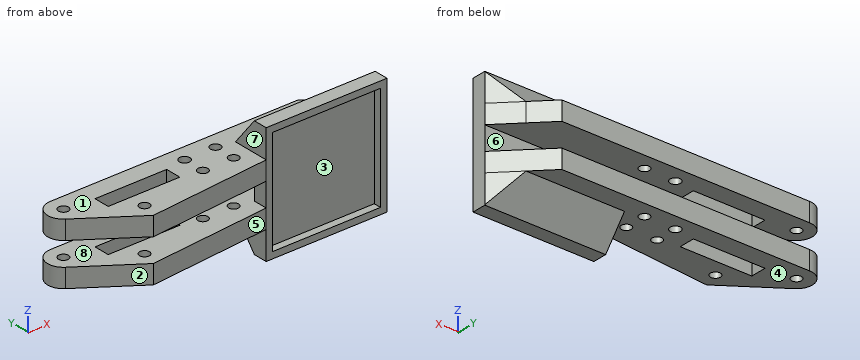
```python
from build123d import *

# Parameters (mm, degrees)
RESSALTO_EXTRUS_O1_DEPTH         = 8
RESSALTO_EXTRUS_O2_DEPTH         = 51.268117765
CORTE_EXTRUS_O1_DEPTH            = 8.000000002
ESBO_O4_W                        = 51.268117776
ESBO_O4_H                        = 10.000000011
CORTE_EXTRUS_O2_DEPTH            = 17.723100001
CORTE_EXTRUS_O3_DEPTH            = 40.852574409
ESBO_O6_W                        = 51.268117776
ESBO_O6_H                        = 10.000000011
CORTE_EXTRUS_O4_DEPTH            = 0.151992449
RESSALTO_EXTRUS_O3_START         = 7.999999998
RESSALTO_EXTRUS_O3_DEPTH         = 7.999999998
RESSALTO_EXTRUS_O4_DEPTH         = 12.017232655
RESSALTO_EXTRUS_O5_DEPTH         = 12.017232657
ESBO_O10_W                       = 30.391419991
ESBO_O10_H                       = 6.689959998
CORTE_EXTRUS_O5_DEPTH            = 135.855194678
ESBO_O11_W                       = 30.391419991
ESBO_O11_H                       = 6.689959998
CORTE_EXTRUS_O6_DEPTH            = 135.855194677
ESBO_O12_W                       = 45.768117767
ESBO_O12_H                       = 44.53446532
CORTE_EXTRUS_O7_DEPTH            = 3.15
INCLINA_O1_START                 = 9.762479363
INCLINA_O1_DEPTH                 = 8.237520637
INCLINA_O2_START                 = -6.465378083
INCLINA_O2_DEPTH                 = 8.465378083
INCLINA_O3_ANGLE                 = 84.752120974
FURO_COM_FOLGA_DE_M41_D          = 4.452840696
FURO_COM_FOLGA_DE_M41_DEPTH      = 7.999999998
FURO_DE_DI_METRO_4_2_4_2_1_D     = 4.2
FURO_DE_DI_METRO_4_2_4_2_1_DEPTH = 7.999999998
FURO_COM_FOLGA_DE_M42_D          = 4.452840696
FURO_COM_FOLGA_DE_M42_DEPTH      = 38.017232657
FURO1_D                          = 4.246430182
FURO1_DEPTH                      = 38.017232657


with BuildPart() as part:
    # Esboço1 → Ressalto-extrusão1 (new body)
    with BuildSketch(Plane.XY.offset(8)):
        with BuildLine():
            Line((-36.110267765, -64.727666859), (-36.110267765, 0))
            Line((-36.110267765, 0), (-107.75607805, 0))
            ThreePointArc((-107.75607805, 0), (-114.12766225, -4.677735132), (-111.573397577, -12.157977319))
            Line((-111.573397577, -12.157977319), (-36.110267765, -64.727666859))
        make_face()
    extrude(amount=-RESSALTO_EXTRUS_O1_DEPTH)

    # Esboço2 → Ressalto-extrusão2 (add)
    with BuildSketch(Plane(origin=(-36.110267765, 0, 0), x_dir=(0, 0, -1), z_dir=(1, 0, 0))):
        with BuildLine():
            Line((2e-09, 1e-09), (2e-09, -23.87509245))
            add(Edge.make_bspline(
                [(2e-09, -64.727666859), (2e-09, -51.110142056), (2e-09, -37.492617253), (2e-09, -23.87509245)],
                knots=[0, 0, 0, 0, 1, 1, 1, 1], degree=3))
            Line((2e-09, -64.727666859), (-18.000000002, -64.727666859))
            add(Edge.make_bspline(
                [(-18.000000002, -64.727666859), (-18.000000002, -51.110142056), (-18.000000002, -37.492617253), (-18.000000002, -23.87509245)],
                knots=[0, 0, 0, 0, 1, 1, 1, 1], degree=3))
            Line((-18.000000002, -23.87509245), (-18.000000002, -17.875092449))
            add(Edge.make_bspline(
                [(-18.000000002, -17.723099999), (-18.000000002, -17.773764149), (-18.000000002, -17.824428299), (-18.000000002, -17.875092449)],
                knots=[0, 0, 0, 0, 1, 1, 1, 1], degree=3))
            add(Edge.make_bspline(
                [(-18.000000002, 1e-09), (-18.000000002, -5.907699999), (-18.000000002, -11.815399999), (-18.000000002, -17.723099999)],
                knots=[0, 0, 0, 0, 1, 1, 1, 1], degree=3))
            Line((-18.000000002, 1e-09), (2e-09, 1e-09))
        make_face()
    extrude(amount=RESSALTO_EXTRUS_O2_DEPTH)

    # Esboço3 → Corte-extrusão1 (cut)
    with BuildSketch(Plane(origin=(0, 0, 0), x_dir=(-1, 0, 0), z_dir=(0, 0, -1))):
        Polygon((-15.15785, 0), (-15.15785, -17.7231), (2.585682, 0), align=None)
    extrude(amount=-CORTE_EXTRUS_O1_DEPTH, mode=Mode.SUBTRACT)

    # Esboço4 → Corte-extrusão2 (cut)
    with BuildSketch(Plane(origin=(0, 0, 0), x_dir=(-1, 0, 0), z_dir=(0, 1, 0))):
        with Locations((10.476208888, 13.000000002)):
            Rectangle(ESBO_O4_W, ESBO_O4_H)
    extrude(amount=-CORTE_EXTRUS_O2_DEPTH, mode=Mode.SUBTRACT)

    # Esboço5 → Corte-extrusão3 (cut)
    with BuildSketch(Plane.XZ.offset(64.727666859)):
        Polygon((15.15785, 18.000000002), (-36.110267765, 18.000000002), (-36.110267765, 8), (-36.110267765, -2e-09), (15.15785, -2e-09), align=None)
    extrude(amount=-CORTE_EXTRUS_O3_DEPTH, mode=Mode.SUBTRACT)

    # Esboço6 → Corte-extrusão4 (cut)
    with BuildSketch(Plane(origin=(0, -17.723100001, 0), x_dir=(-1, 0, 0), z_dir=(0, 1, 0))):
        with Locations((10.476208888, 13.000000002)):
            Rectangle(ESBO_O6_W, ESBO_O6_H)
    extrude(amount=-CORTE_EXTRUS_O4_DEPTH, mode=Mode.SUBTRACT)

    # Esboço7 → Ressalto-extrusão3 (add)
    with BuildSketch(Plane.XY.offset(18.000000002).offset(RESSALTO_EXTRUS_O3_START)):
        with BuildLine():
            Line((-36.110267767, -23.87509245), (-36.110267767, -64.727666793))
            Line((-36.110267767, -64.727666793), (-111.573397573, -12.157977315))
            ThreePointArc((-111.573397573, -12.157977315), (-114.127662248, -4.677735132), (-107.75607805, 1e-09))
            Line((-107.75607805, 1e-09), (-2.585681995, 1e-09))
            Line((-2.585681995, 1e-09), (5.698950337, -8.275092449))
            Line((5.698950337, -8.275092449), (15.157849978, -17.723100021))
            Line((15.157849978, -17.723100021), (15.157849978, -23.87509245))
            Line((15.157849978, -23.87509245), (-36.110267767, -23.87509245))
        make_face()
    extrude(amount=-RESSALTO_EXTRUS_O3_DEPTH)

    # Esboço8 → Ressalto-extrusão4 (add)
    with BuildSketch(Plane(origin=(0, 0, 0), x_dir=(-1, 0, 0), z_dir=(0, 0, -1))):
        Polygon((36.110267765, -8.275092449), (36.110267765, -23.87509245), (-15.15785, -23.87509245), (-15.15785, -17.7231), (-5.698950354, -8.275092449), align=None)
    extrude(amount=RESSALTO_EXTRUS_O4_DEPTH)

    # Esboço9 → Ressalto-extrusão5 (add)
    with BuildSketch(Plane.XY.offset(26)):
        Polygon((15.15785, -17.7231), (15.15785, -23.87509245), (-36.110267765, -23.87509245), (-36.110267765, -8.275092449), (5.698950354, -8.275092449), align=None)
    extrude(amount=RESSALTO_EXTRUS_O5_DEPTH)

    # Esboço10 → Corte-extrusão5 (cut, through all)
    with BuildSketch(Plane.XY.offset(8)):
        with Locations((-80.248070001, -11.317270001)):
            Rectangle(ESBO_O10_W, ESBO_O10_H)
    extrude(amount=-CORTE_EXTRUS_O5_DEPTH, mode=Mode.SUBTRACT)

    # Esboço11 → Corte-extrusão6 (cut, through all)
    with BuildSketch(Plane(origin=(0, 0, 18.000000002), x_dir=(-1, 0, 0), z_dir=(0, 0, -1))):
        with Locations((80.248070001, -11.317270001)):
            Rectangle(ESBO_O11_W, ESBO_O11_H)
    extrude(amount=-CORTE_EXTRUS_O6_DEPTH, mode=Mode.SUBTRACT)

    # Esboço12 → Corte-extrusão7 (cut)
    with BuildSketch(Plane.XZ.offset(23.87509245)):
        with Locations((-10.476208882, 13)):
            Rectangle(ESBO_O12_W, ESBO_O12_H)
    extrude(amount=-CORTE_EXTRUS_O7_DEPTH, mode=Mode.SUBTRACT)

    # Inclinação1: read off the stored shape, not the designer's step
    # Inclinação1 outline → Inclinação1 (cut)
    with BuildSketch(Plane(origin=(0, 0, 0), x_dir=(1, 0, 0), z_dir=(0, 0.7813058431702609, 0.624148363314371)).offset(INCLINA_O1_START)):
        Polygon((-36.110267765, -40.859795712), (15.15785, -40.859795712), (15.15785, -40.616276003), (5.698950337, -25.478837331), (-36.110267765, -25.478837331), align=None)
    extrude(amount=INCLINA_O1_DEPTH, mode=Mode.SUBTRACT)

    # Inclinação2: read off the stored shape, not the designer's step
    # Inclinação2 outline → Inclinação2 (cut)
    with BuildSketch(Plane(origin=(0, 0, 0), x_dir=(1, 0, 0), z_dir=(0, 0.7813058431702609, -0.624148363314371)).offset(INCLINA_O2_START)):
        Polygon((5.698950354, 5.164885408), (15.15785, 20.302324047), (15.15785, 20.545843787), (-36.110267765, 20.545843787), (-36.110267765, 5.164885408), align=None)
    extrude(amount=INCLINA_O2_DEPTH, mode=Mode.SUBTRACT)

    # Inclinação3
    inclina_o3_faces = [part.faces().sort_by_distance(p)[0] for p in [
        (-36.110267765, -44.301379654, 3.999999999),
        (-36.110267767, -44.301379621, 22.000000001),
    ]]
    draft(inclina_o3_faces, Plane(origin=(0, -23.87509245, 0), x_dir=(0, 0, -1), z_dir=(0, -1, 0)), INCLINA_O3_ANGLE)

    # Furo com folga de M41
    with Locations(Plane.XY.offset(26)):
        with Locations((-56.444514416, -6.798608997)):
            Hole(FURO_COM_FOLGA_DE_M41_D / 2, depth=FURO_COM_FOLGA_DE_M41_DEPTH)

    # Furo de diâmetro Ø4.2 (4.2)1
    with Locations(Plane.XY.offset(26)):
        with Locations((-85.990622049, -21.806552958), (-107.75607805, -6.678263028), (-43.350632153, -6.798608997), (-56.444514416, -16.052089875), (-43.350632153, -16.052089875)):
            Hole(FURO_DE_DI_METRO_4_2_4_2_1_D / 2, depth=FURO_DE_DI_METRO_4_2_4_2_1_DEPTH)

    # Furo com folga de M42
    with Locations(Plane(origin=(0, 0, 0), x_dir=(-1, 0, 0), z_dir=(0, 0, -1))):
        with Locations((56.444514416, -6.798608997)):
            Hole(FURO_COM_FOLGA_DE_M42_D / 2, depth=FURO_COM_FOLGA_DE_M42_DEPTH)

    # Furo1
    with Locations(Plane(origin=(0, 0, 0), x_dir=(-1, 0, 0), z_dir=(0, 0, -1))):
        with Locations((43.350632153, -16.052089875), (56.444514416, -16.052089875), (43.350632153, -6.798608997), (107.75607805, -6.678263028), (85.990622049, -21.806552958)):
            Hole(FURO1_D / 2, depth=FURO1_DEPTH)


solid = part.part
```
Could you check a few things on this model? Use its own coordinates, in mm. Face numbers are marked on the shaded views. A direction names the side the tool comes from. Coordinates: 2 decimals unless noted, no trailing zeros. Write each loop counter-clockwise with the first axis right and the second up, starting at its lowest first coordinate (ties: lowest second). Pieces come first, ordered by that corner, then holes. Notation, with made-up numbers: M 87,50 L 138,50 A24 ccw 138,74 Z; hole C -1.75,25 d4. An arc over 180 degrees is marked long. Answer as CSV lines item,"result". Start each with the question number.
1) We'd pull the mould along Z, two halves only. Please class the marked faces 1, 2, 3 and 4: +Z half, -Z half, draft (parallel to the pull), parting line (faces both ways), or undercut.
2) For P1, Ø10, axis at y = -5.5, z = 3, coming from the +X side; P2, Ø5, axis at y = -21.5, z = 15, coming from the -X side; P3, Ø4, axis at x = -92, y = -3.5, coming from the +Z side, each with a flat end and sliding along its axis, tell me the tip position at first contact or that it passes through.
3) I want a section at B-B, the plane y = -10.5. Please give me the cut outline in (x, z).
4) Please list where these lines run through material, in increasing order: line 1 (Z direction, x = -81, y = -7.5); line 2 (X direction, y = -23.5, z = 9); line 3 (X direction, y = -22.75, z = 22). Write a range as from..to.
5) I want a section at C-C, the plane x = -31.5. Please give me the cut outline in (y, z), and give its area (3 significant figures).
6) I want a section at D-D, the plane z = 15.5. Please give me the cut outline in (x, y).
7) For the marked faces 5, 6, 7 and 8, which set-ups out of +Z, -Z, +X, -X, +Y, -Y let a thin tool reach every point of the face, with its end or its side?
8) I want a section at A-A, the plane x = -70.5. Please give me the cut outline in (y, z), and give its area (3 significant figures).
Data:
1,face 1,"+Z half"
1,face 2,"draft"
1,face 3,"undercut"
1,face 4,"-Z half"
2,P1,"stops at x = 7.93"
2,P2,"stops at x = -36.11"
2,P3,"stops at z = 26"
3,outline,"M -113.23,0 L -95.44,0 L -95.44,8 L -113.23,8 Z; M -113.23,18 L -95.44,18 L -95.44,26 L -113.23,26 Z; M -65.05,0 L -36.11,0 L -36.11,-2.79 L 7.93,-2.79 L 7.93,8 L -65.05,8 Z; M -65.05,18 L 7.93,18 L 7.93,28.79 L -36.11,28.79 L -36.11,26 L -65.05,26 Z"
4,line 1,"z = 0..8, 18..26"
4,line 2,"x = -36.11..-33.36, 12.41..15.16"
4,line 3,"x = -96.37..-87.89, -84.09..-33.36, 12.41..15.16"
5,outline,"M -23.88,-12.02 L -17.88,-12.02 L -8.28,0 L 0,0 L 0,8 L -17.88,8 L -17.88,18 L 0,18 L 0,26 L -8.28,26 L -17.88,38.02 L -23.88,38.02 L -23.88,35.27 L -20.73,35.27 L -20.73,-9.27 L -23.88,-9.27 Z"
5,area,"561 mm^2"
6,outline,"M -36.11,-23.88 L -33.36,-23.88 L -33.36,-20.73 L 12.41,-20.73 L 12.41,-23.88 L 15.16,-23.88 L 15.16,-17.88 L -36.11,-17.88 Z"
7,face 5,"+Z, -Z, +X, -Y"
7,face 6,"+X, -X, +Y"
7,face 7,"+Z, -X, +Y, -Y"
7,face 8,"-X, +Y"
8,outline,"M -27.03,0 L -14.66,0 L -14.66,8 L -27.03,8 Z; M -27.03,18 L -14.66,18 L -14.66,26 L -27.03,26 Z; M -7.97,0 L 0,0 L 0,8 L -7.97,8 Z; M -7.97,18 L 0,18 L 0,26 L -7.97,26 Z"
8,area,"326 mm^2"
